Input: part model. Units: mm. Frame: model coordinates. Coordinates: 2 decimals unless noted, no trailing zeros. Loops run counter-clockwise (first coordinate to the right, second up) from the corner with the lowest first, then second, coordinate; pieces in that order, holes last.
```python
from build123d import *

# Parameters (mm, degrees)
F1_DEPTH  = 3
F3_DEPTH  = 25
F4_R      = 5
F5_R      = 11.15
F5_R_2    = 2.65
F6_DEPTH  = 25
F7_W      = 78
F7_H      = 55.5
F7_R      = 2
F8_DEPTH  = 25
F9_R      = 8.15
F10_DEPTH = 25


with BuildPart() as f1:
    # F0 (on Top) → F1 (new body)
    with BuildSketch(Plane.XY):
        with BuildLine():
            Line((-197.8147600734, 20.7911690818), (-202.2340594865, 0))
            Line((-202.2340594865, 0), (216.0975214603, 0))
            Line((216.0975214603, 0), (209.2885731253, 20.7911690818))
            ThreePointArc((209.2885731253, 20.7911690818), (167.4870934164, 78.1154778874), (100, 100))
            Line((100, 100), (-100, 100))
            ThreePointArc((-100, 100), (-162.932039105, 77.7145961457), (-197.8147600734, 20.7911690818))
        make_face()
    extrude(amount=F1_DEPTH)

    # F2 (on face) → F3 (cut)
    with BuildSketch(Plane.XY.offset(3)):
        with BuildLine():
            ThreePointArc((1.5842979518, 0), (9.4530988092, 4.1693984068), (12.6, 12.5))
            ThreePointArc((12.6, 12.5), (12.2192388124, 15.5741182224), (11.0999678023, 18.4624420155))
            ThreePointArc((11.0999678023, 18.4624420155), (0, 25.1), (-11.0999678023, 18.4624420155))
            ThreePointArc((-11.0999678023, 18.4624420155), (-11.1999147641, 6.7274867453), (-1.5842979518, 0))
            Line((-1.5842979518, 0), (1.5842979518, 0))
        make_face()
        with BuildLine():
            ThreePointArc((11.0999678023, 18.4624420155), (12.2192388124, 15.5741182224), (12.6, 12.5))
            ThreePointArc((12.6, 12.5), (9.4530988092, 4.1693984068), (1.5842979518, 0))
            Line((1.5842979518, 0), (21.7592636698, 0))
            Line((21.7592636698, 0), (11.0999678023, 18.4624420155))
        make_face()
        with BuildLine():
            ThreePointArc((-1.5842979518, 0), (0, -0.1), (1.5842979518, 0))
            Line((1.5842979518, 0), (-1.5842979518, 0))
        make_face()
        with BuildLine():
            ThreePointArc((-1.5842979518, 0), (-11.1999147641, 6.7274867453), (-11.0999678023, 18.4624420155))
            Line((-11.0999678023, 18.4624420155), (-21.7592636698, 0))
            Line((-21.7592636698, 0), (-1.5842979518, 0))
        make_face()
    extrude(amount=-F3_DEPTH, mode=Mode.SUBTRACT)

    # F4
    f4_edges = [f1.edges().sort_by_distance(p)[0] for p in [
        (-21.759264, 0, 1.5),
        (21.759264, 0, 1.5),
    ]]
    fillet(f4_edges, radius=F4_R)

    # F5 (on face) → F6 (cut)
    with BuildSketch(Plane.XY.offset(3)):
        Polygon((-145, 38.9489291724), (-152.75, 34.4744645862), (-152.75, 25.5255354138), (-145, 21.0510708276), (-137.25, 25.5255354138), (-137.25, 34.4744645862), align=None)
        with Locations((-115, 30)):
            Circle(F5_R)
        with Locations((-115, 60)):
            Circle(F5_R_2)
        with Locations((-145, 60)):
            Circle(F5_R_2)
    extrude(amount=-F6_DEPTH, mode=Mode.SUBTRACT)

    # F7 (on face) → F8 (cut)
    with BuildSketch(Plane.XY.offset(3)):
        with Locations((0, 57.75)):
            Rectangle(F7_W, F7_H)
        with Locations((-42.6313167033, 28.25)):
            Circle(F7_R)
        with Locations((-42.6313167033, 87.25)):
            Circle(F7_R)
        with Locations((42.3686832967, 87.25)):
            Circle(F7_R)
        with Locations((42.3686832967, 28.25)):
            Circle(F7_R)
    extrude(amount=-F8_DEPTH, mode=Mode.SUBTRACT)

    # F9 (on face) → F10 (cut)
    with BuildSketch(Plane.XY.offset(3)):
        with Locations((115, 30)):
            Circle(F9_R)
    extrude(amount=-F10_DEPTH, mode=Mode.SUBTRACT)


solid = f1.part
```
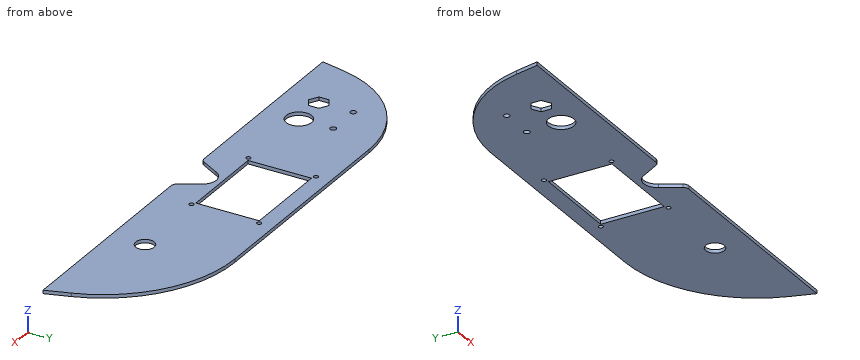
Item 1: Contact query for flat-ended pins moving along their axis: P1, Ø6.5, axis at x = 42.37, y = 87.25, coming from the +Z side; P2, Ø1.5, axis at y = 30, z = 2, coming from the -X side; P3, Ø1.5, axis at x = 6, z = 2, coming from the -Y side; P4, Ø0.9, axis at y = 54, z = 1, coming from the +X side. Output: stop coordinate, or through.
Result:
P1: stops at z = 3
P2: stops at x = -195.63
P3: stops at y = 23.14
P4: stops at x = 192.34
Item 2: Section query A-A (z = 1.7). Count the separate pieces of the cut face and the enclosed holes in it, then the cut area to 3 significant figures.
Result:
separate pieces: 1
enclosed holes: 10
area: 30,600 mm2
Item 3: Line query: L1, parallel to Y at x = -43, z = 2.1; L2, parallel to X at y = 21, z = 0.75; L3, parallel to X at y = 23, z = 1.7. Output: solid intervals per line, ascending.
Result:
L1: y = 0 to 26.28, 30.22 to 85.28, 89.22 to 100
L2: x = -197.77 to -121.58, -108.42 to -9.3, 9.3 to 209.22
L3: x = -197.32 to -148.38, -141.62 to -123.68, -106.32 to -6.96, 6.96 to 110.83, 119.17 to 208.54
Item 4: Section query C-C (x = 154.5). Output: boundary loops of the cut face in (y, z).
Result:
outline: (0, 0) - (86.27, 0) - (86.27, 3) - (0, 3) - close
Item 5: Section query B-B (y = 7.5). Output: boundary loops of the cut face in (x, z).
Result:
outline: (-200.64, 0) - (-17.43, 0) - (-17.43, 3) - (-200.64, 3) - close; (17.43, 0) - (213.64, 0) - (213.64, 3) - (17.43, 3) - close
